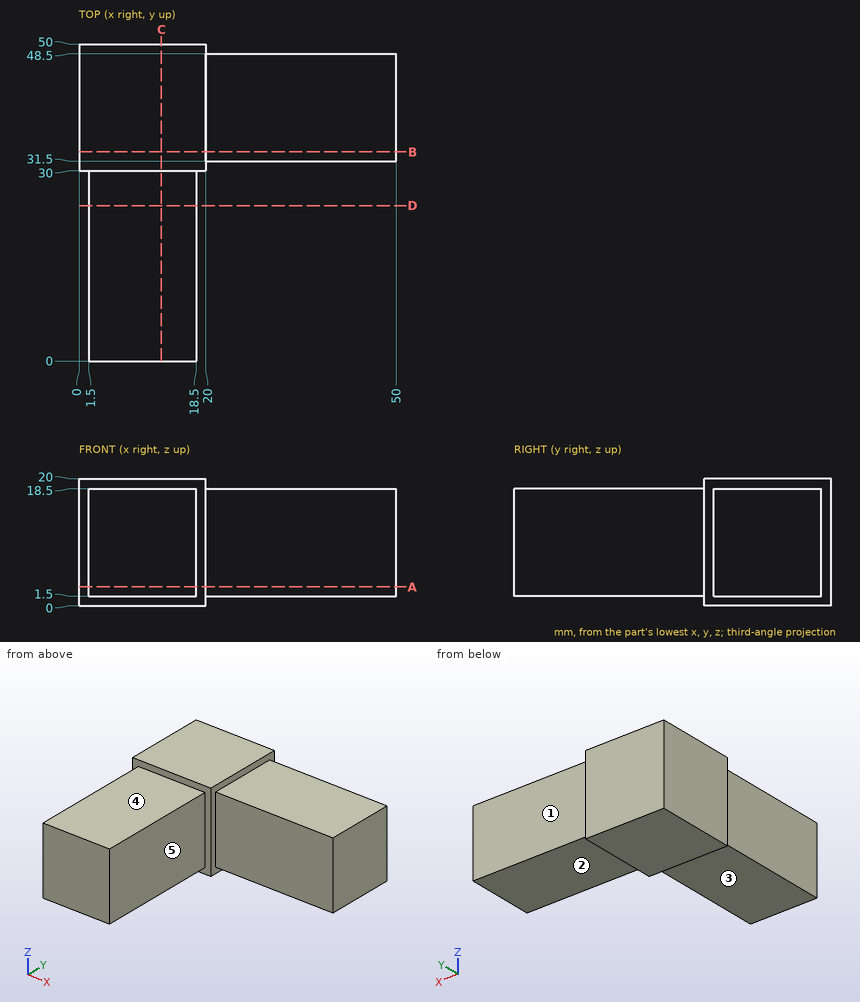
Could you check a few things on this drawing? It's one solid part, dimensions in mm from its lowest x, y, z. A direction names the side the tool comes from. Round coordinates to 2 decimals unless told otherwise and drop trailing zeros. Write each loop counter-clockwise with the first axis right and the second up, starting at its lowest first coordinate (ties: lowest second). Pieces come first, ordered by that corner, then holes. Notation, with made-up numbers: (69.25, 52) -> (120.25, 52) arc R25 ccw to (120.25, 85) -> close; hole circle Ø9 at (-16.5, 13). An arc over 180 degrees is marked (long way). Use one line per item in the form item = value. Start each with the question number.
Q1. I'm going to push flat-ended pins straight in: P1, Ø4, axis at x = 33.5, z = 6, coming from the -Y side; P2, Ø5, axis at x = 36, y = 40.5, coming from the -Z side; P3, Ø12, axis at x = 18.5, z = 12, coming from the -Y side; P4, Ø8.5, axis at y = 22, z = 6.5, coming from the -X side. Where does each tip first touch, or does it pass through?
Q2. If I drill on probe 1 along Y at (x, z) = (30, 4.5); probe 2 along Z at (x, y) = (26.5, 46); probe 3 along Y at (x, z) = (6.5, 19), over which ranges is the centre line in solid material (lowest first)? Write a range as [from, to].
Q3. Imagine slicing it at B-B (y = 33). Please give me the cut outline in (x, z), then the cut area to 3 significant figures.
Q4. Imagine slicing it at A-A (z = 3). Please give me the cut outline in (x, y).
Q5. Imagine slicing it at C-C (x = 13). Please give me the cut outline in (y, z).
Q6. Imagine slicing it at D-D (y = 24.5). Please give me the cut outline in (x, z), then the cut area to 3 significant figures.
Q7. Which directions (+Z, -Z, +X, -X, +Y, -Y) give clear straight access to the entire face, cutting with the end or side of a thin tool? Please do the marked faces 1, 2, 3, 4 and 5.
Worked out:
q1.P1 = 31.5
q1.P2 = 1.5
q1.P3 = 0
q1.P4 = 1.5
q2.probe_1 = [31.5, 48.5]
q2.probe_2 = [1.5, 18.5]
q2.probe_3 = [30, 50]
q3.outline = (0, 0) -> (20, 0) -> (20, 1.5) -> (50, 1.5) -> (50, 18.5) -> (20, 18.5) -> (20, 20) -> (0, 20) -> close
q3.area = 910 mm^2
q4.outline = (0, 30) -> (1.5, 30) -> (1.5, 0) -> (18.5, 0) -> (18.5, 30) -> (20, 30) -> (20, 31.5) -> (50, 31.5) -> (50, 48.5) -> (20, 48.5) -> (20, 50) -> (0, 50) -> close
q5.outline = (0, 1.5) -> (30, 1.5) -> (30, 0) -> (50, 0) -> (50, 20) -> (30, 20) -> (30, 18.5) -> (0, 18.5) -> close
q6.outline = (1.5, 1.5) -> (18.5, 1.5) -> (18.5, 18.5) -> (1.5, 18.5) -> close
q6.area = 289 mm^2
q7.face_1 = +Z, -Z, +X, +Y
q7.face_2 = -Z, +X, +Y, -Y
q7.face_3 = -Z, +X, -X, -Y
q7.face_4 = +Z, +X, -X, -Y
q7.face_5 = +Z, -Z, +X, -Y
